Autodesk Inventor part; units mm, degrees
ref_plane "YZ Plane" through (0, 0, 0) normal (1, 0, 0) x (0, 1, 0)
ref_plane "XZ Plane" through (0, 0, 0) normal (0, 1, 0) x (-1, 0, 0)
ref_plane "XY Plane" through (0, 0, 0) normal (0, 0, 1) x (1, 0, 0)
sketch "Sketch1" plane through (0, 0, 0) normal (1, 0, 0) x (0, 1, 0)
  line L0 (1620, 0) -> (70, 0)
  line L1 (70, 0) -> (20, 0)
  line L2 (20, 0) -> (0, 0)
  dimension "d0" = 180
  dimension "d1" = 50
  dimension "d2" = 1620
  dimension "d3" = 20
contour flange "Contour Flange1" sketch "Sketch1" thickness 3 bend radius 3 width 1200 along (1, 0, 0) mid plane no both sides no wall seen from (0, 845, 0) lies toward (0, 0, 1) curves L0 L1
bend "Bend1"
corner "Corner1"
sketch "Sketch3" plane through (0, 49.7046, 0) normal (0, 0, -1) x (-1, 0, 0)
  line L0 (-1197.5147, 1570.2954) -> (-1197.5147, -29.7046) construction
  line L1 (0, 1570.2954) -> (0, -29.7046)
  line L2 (-1200, 1570.2954) -> (0, 1570.2954) construction
  line L3 (0, 1570.2954) -> (0, -29.7046)
  circle A0 centre (0, 1070.2954) radius 213
  line L4 (0, -29.7046) -> (-1200, -29.7046)
  point P0 (0, -49.7046)
  point P1 (0, 0)
  point P2 (0, 857.2954)
  point P3 (0, 1283.2954)
  dimension "d25" = 426
  dimension "d26" = 500
extrude "Cut1" cut sketch "Sketch3" against normal blind 3 contours L1 A0 picked at (-58.5713, 1129.0628)
sketch "Sketch2" plane through (1197.8787, 20, 0.8787) normal (0.7071068, 0, 0.7071068) x (0, 1, 0)
  line L0 (1600, 0) -> (0, 0)
  line L1 (0, 0) -> (0, -50)
  line L2 (0, -50) -> (1600, -50)
  line L3 (1600, -50) -> (1600, 0)
equation "\"d27\" = Thickness"
equation "\"d4\" = Thickness"
equation "\"d5\" = BendReliefWidth"
equation "\"d6\" = BendReliefDepth"
equation "\"d7\" = MinimumRemnant"
equation "\"d8\" = TransitionRadius"
equation "\"d10\" = BendRadius"
equation "\"d12\" = CornerReliefSize"
equation "\"d13\" = GapSize"
equation "\"d14\" = JacobiRadiusSize"
equation "\"BendRadius\" = Thickness"
equation "\"BendReliefWidth\" = Thickness"
equation "\"BendReliefDepth\" = 0.5 * Thickness"
equation "\"CornerReliefSize\" = 4 * Thickness"
equation "\"MinimumRemnant\" = 2 * Thickness"
equation "\"TransitionRadius\" = BendRadius"
equation "\"JacobiRadiusSize\" = BendRadius"
equation "\"GapSize\" = Thickness"
properties part number "GBK-RK-0017 long wall 3"
Here's how the part is built. I have some questions about the finished solid (model axes, mm). Give positions to 0.01 mm unless a question says otherwise; leave off trailing zeros. Order: outer loops, then holes, each group sorted by start corner. A loop starts at its lowest first (then second) coordinate and runs counter-clockwise, first axis right, second up. Notation, with made-up numbers: (-7.75, 62) -> (7.25, 62) arc R16 ccw to (7.25, 80) -> close; hole circle Ø5 at (-15, 88.25). An arc over 180 degrees is marked (long way). Use a Markdown table: item, result. Add a question column.
Item 1: Imagine slicing it at C-C on y = 1120. Please give me the cut outline in (x, z).
Item 2: Imagine slicing it at A-A on x = 116. Please give me the cut outline in (y, z).
Item 3: Imagine slicing it at B-B on z = 0.55. Please give me the cut outline in (x, y), plus the area to 3 significant figures.
Item 4: I need wall thicknesses on line 1 (Y direction, x = 138, z = 1.05); line 2 (X direction, y = 1208.5, z = 2.4); line 3 (X direction, y = 1008.5, z = 0.35). Which ranges of each line are inside material? Lowest first, please.
Data:
| question | item | result |
|---|---|---|
| 1 | outline | (213, 0) -> (1200, 0) -> (1200, 3) -> (213, 3) -> close |
| 2 | outline | (20, 0) -> (941.36, 0) -> (941.36, 3) -> (20, 3) -> close; (1298.64, 0) -> (1620, 0) -> (1620, 3) -> (1298.64, 3) -> close |
| 3 | outline | (0, 20) -> (1200, 20) -> (1200, 1620) -> (0, 1620) -> (0, 1333) arc R213 cw to (0, 907) -> close |
| 3 | area | 1,850,000 mm² |
| 4 | line 1 | y = 20 to 957.75, 1282.25 to 1620 |
| 4 | line 2 | x = 193.74 to 1200 |
| 4 | line 3 | x = 181.48 to 1200 |
